Design review of the part built by this model. Coordinates are the model's own, in mm. A direction names the side the tool comes from. Round coordinates to 2 decimals unless told otherwise and drop trailing zeros. Order: outer loops, then holes, each group sorted by start corner. A loop starts at its lowest first (then second) coordinate and runs counter-clockwise, first axis right, second up. Notation, with made-up numbers: M -3.75,-16 L 3.25,-16 A20 ccw 3.25,20 Z; hole C 27.5,12.25 d4. An arc over 180 degrees is marked long. Use a Markdown table: item, result. Add a question column.
(1) Take a section at A-A (z = 31). Write out the cut boundary in (x, y).
(2) For pin 1 (1 mm diameter, centred on x = -4, z = 34.5, fed in from -Y); pin 2 (5.5 mm diameter, centred on y = 0.5, z = 26.5, fed in from +X); pin 3 (1.2 mm diameter, centred on x = 12, z = 22.5, fed in from -Y); pin 4 (1 mm diameter, centred on y = 14, z = 21.5, fed in from +X), all flat-tipped, find the tip position at first contact; note any pin that passes through.
(3) Take a section at B-B (z = -4). Write out the cut boundary in (x, y).
(4) Machinability: for faces 4 (the face through (13, 0, 0)), 5 (the face through (12, -2.5, 21)), 6 (the face through (-8.43, 6.54, 42)), which of the approach directions +Z, -Z, +X, -X, +Y, -Y give a long, thin tool a straight path to every point of the face, cutting with its end or side? Answer none if there is none.
(5) To check wall thickness, follow probe 1 along Z at (x, y) = (2, -1); probe 2 along X at (y, z) = (-4, 16); probe 3 along Y at (x, z) = (-3, 18.5). State the ranges of each line that lie inside material, in increasing order. Write a range as from..to.
(6) The part is to be moulded in two halves that separate along X. For faces 1 (the face through (0, 0, 0)), 2 (the face through (11.247, 0, 21)), 3 (the face through (12, 2.5, 21)), say which applies: released by +X, released by -X, zero draft, split by the parting line, or undercut.
```python
from build123d import *

# Parameters (mm, degrees)
F0_W     = 38.7298334621
F0_H     = 10
F1_DEPTH = 10
F3_DEPTH = 42
F4_R     = 0.5


with BuildPart() as f1:
    # F0 (on Top) → F1 (new body)
    with BuildSketch(Plane.XY):
        with BuildLine():
            Line((-19.364916731, 5), (19.364916731, 5))
            ThreePointArc((19.364916731, 5), (0, 20), (-19.364916731, 5))
        make_face()
        with BuildLine():
            Line((-19.364916731, -5), (-19.364916731, 5))
            ThreePointArc((-19.364916731, 5), (-20, 0), (-19.364916731, -5))
        make_face()
        with BuildLine():
            ThreePointArc((-19.364916731, -5), (0, -20), (19.364916731, -5))
            Line((19.364916731, -5), (-19.364916731, -5))
        make_face()
        Rectangle(F0_W, F0_H)
    extrude(amount=-F1_DEPTH)

    # F2 (on face) → F3 (join)
    with BuildSketch(Plane.XY):
        with BuildLine():
            Line((11.2474487139, 2.5), (12.2474487139, 2.5))
            ThreePointArc((12.2474487139, 2.5), (0, 12.5), (-12.2474487139, 2.5))
            Line((-12.2474487139, 2.5), (-9.6824583655, 2.5))
            ThreePointArc((-9.6824583655, 2.5), (0, 10), (9.6824583655, 2.5))
            Line((9.6824583655, 2.5), (11.2474487139, 2.5))
        make_face()
        with BuildLine():
            Line((11.2474487139, -2.5), (11.2474487139, 2.5))
            Line((11.2474487139, 2.5), (9.6824583655, 2.5))
            ThreePointArc((9.6824583655, 2.5), (9.9202969627, 1.2600429248), (10, 0))
            ThreePointArc((10, 0), (9.9202969627, -1.2600429248), (9.6824583655, -2.5))
            Line((9.6824583655, -2.5), (11.2474487139, -2.5))
        make_face()
        with BuildLine():
            ThreePointArc((-12.2474487139, -2.5), (0, -12.5), (12.2474487139, -2.5))
            Line((12.2474487139, -2.5), (11.2474487139, -2.5))
            Line((11.2474487139, -2.5), (9.6824583655, -2.5))
            ThreePointArc((9.6824583655, -2.5), (0, -10), (-9.6824583655, -2.5))
            Line((-9.6824583655, -2.5), (-12.2474487139, -2.5))
        make_face()
        with BuildLine():
            Line((-9.6824583655, 2.5), (-12.2474487139, 2.5))
            Line((-12.2474487139, 2.5), (-12.2474487139, -2.5))
            Line((-12.2474487139, -2.5), (-9.6824583655, -2.5))
            ThreePointArc((-9.6824583655, -2.5), (-10, 0), (-9.6824583655, 2.5))
        make_face()
        with BuildLine():
            Line((-12.2474487139, -2.5), (-12.2474487139, 2.5))
            ThreePointArc((-12.2474487139, 2.5), (-12.5, 0), (-12.2474487139, -2.5))
        make_face()
    extrude(amount=F3_DEPTH)

    # F4
    f4_edges = [f1.edges().sort_by_distance(p)[0] for p in [
        (9.682458, 2.5, 42),
        (-12.5, 0, 0),
        (-20, 0, 0),
    ]]
    fillet(f4_edges, radius=F4_R)


solid = f1.part
```
Verdict:
| question | item | result |
|---|---|---|
| 1 | outline | M 11.25,-2.5 L 11.25,2.5 L 12.25,2.5 A12.5 ccw long 12.25,-2.5 Z; hole C 0,0 d20 |
| 2 | pin 1 | stops at y = -12 |
| 2 | pin 2 | stops at x = 12.25 |
| 2 | pin 3 | stops at y = -5.13 |
| 2 | pin 4 | passes through |
| 3 | outline | M 19.36,-5 L 19.36,5 A20 ccw long Z |
| 4 | face 4 | +Z |
| 4 | face 5 | +Z, +X |
| 4 | face 6 | +Z, +X, -X, +Y, -Y |
| 5 | probe 1 | z = -10..0 |
| 5 | probe 2 | x = -11.84..-9.17, 9.17..11.84 |
| 5 | probe 3 | y = -12.13..-9.54, 9.54..12.13 |
| 6 | face 1 | undercut |
| 6 | face 2 | released by +X |
| 6 | face 3 | zero draft |
